```python
from build123d import *

# Parameters (mm, degrees)
F0_R     = 1.5
F0_R_2   = 1.65
F0_R_3   = 5
F1_DEPTH = 3
F2_R     = 5


with BuildPart() as f1:
    # F0 (on Top) → F1 (new body)
    with BuildSketch(Plane.XY):
        with BuildLine():
            add(Edge.make_bspline(
                [(-52.118164, 69.593788), (-40.285984, 48.277058), (-22.257566, 29.243172), (0, 20)],
                knots=[9.256523, 9.256523, 9.256523, 9.256523, 80.865454, 80.865454, 80.865454, 80.865454], degree=3))
            ThreePointArc((-52.118164, 69.593788), (-51.973476, 68.388311), (-51.925144, 67.175144))
            ThreePointArc((-51.925144, 67.175144), (-57.28378, 55.568103), (-69.593788, 52.118164))
            add(Edge.make_bspline(
                [(-69.593788, 52.118164), (-48.277057, 40.285984), (-29.243172, 22.257566), (-20, 0)],
                knots=[9.256523, 9.256523, 9.256523, 9.256523, 80.865454, 80.865454, 80.865454, 80.865454], degree=3))
            Line((-20, 0), (0, 0))
            Line((0, 0), (0, 20))
        make_face()
        with Locations((-18, 6.25)):
            Circle(F0_R, mode=Mode.SUBTRACT)
        with Locations((-7.5, 7.5)):
            Circle(F0_R, mode=Mode.SUBTRACT)
        with Locations((-6.25, 18)):
            Circle(F0_R, mode=Mode.SUBTRACT)
        with BuildLine():
            add(Edge.make_bspline(
                [(-56.391766, 77.958523), (-55.0736, 75.142944), (-53.64765, 72.349293), (-52.118164, 69.593788)],
                knots=[0, 0, 0, 0, 9.256523, 9.256523, 9.256523, 9.256523], degree=3))
            ThreePointArc((-56.391766, 77.958523), (-77.958523, 77.958523), (-77.958523, 56.391766))
            add(Edge.make_bspline(
                [(-77.958523, 56.391766), (-75.142944, 55.0736), (-72.349293, 53.647649), (-69.593788, 52.118164)],
                knots=[0, 0, 0, 0, 9.256523, 9.256523, 9.256523, 9.256523], degree=3))
            ThreePointArc((-69.593788, 52.118164), (-57.28378, 55.568103), (-51.925144, 67.175144))
            ThreePointArc((-51.925144, 67.175144), (-51.973476, 68.388311), (-52.118164, 69.593788))
        make_face()
        with Locations((-67.175142, 57.675142)):
            Circle(F0_R_2, mode=Mode.SUBTRACT)
        with Locations((-75.175142, 67.175142)):
            Circle(F0_R_2, mode=Mode.SUBTRACT)
        with Locations((-67.175142, 67.175142)):
            Circle(F0_R_3, mode=Mode.SUBTRACT)
        with Locations((-67.175142, 76.675142)):
            Circle(F0_R_2, mode=Mode.SUBTRACT)
        with Locations((-59.175142, 67.175142)):
            Circle(F0_R_2, mode=Mode.SUBTRACT)
    extrude(amount=F1_DEPTH)

    # F2
    f2_edges = [f1.edges().sort_by_distance(p)[0] for p in [
        (-56.391766, 77.958523, 1.5),
        (-77.958523, 56.391766, 1.5),
    ]]
    fillet(f2_edges, radius=F2_R)


solid = f1.part
```
Model file for the job. Use its own axes, mm. Give positions to 0.01 mm unless a question says otherwise; leave off trailing zeros.
1) Pin check, flat tips, straight feed: pin 1 (4 mm diameter, centred on x = -67.18, y = 57.68, fed in from +Z); pin 2 (1.5 mm diameter, centred on x = -52.5, z = 1, fed in from -Y); pin 3 (1.5 mm diameter, centred on x = -47.5, z = 0.5, fed in from -Y). Stop position of each tip, or through.
2) Saw through at A-A, the plane z = 2.2. Count the separate pieces of the cut face and the enclosed holes in it, then the cut area to 3 significant figures.
3) Mould opens along X. For faces 1 (the cylindrical face through (-68.485, 56.671, 1.479)), 2 (the flat face through (-41, 41, 3)), 3 (the flat face through (0, 10, 1)), 4 (the cylindrical face through (-77.73, 78.18, 1.48)) say: +X half, -X half, draft (parallel to the pull), parting line (faces both ways), or undercut.
4) Wall check: probe 1 along Y at (x, z) = (-58, 2.85); probe 2 along Y at (x, z) = (-74.5, 2.05); probe 3 along X at (y, z) = (76, 0.95). Give the ranges that are in metal, low to high.
Computed:
1. pin 1: stops at z = 3
1. pin 2: stops at y = 40.26
1. pin 3: stops at y = 36.1
2. separate pieces: 1
2. enclosed holes: 8
2. area: 2,000 mm2
3. face 1: undercut
3. face 2: draft
3. face 3: +X half
3. face 4: parting line
4. probe 1: y = 44.9 to 66.02, 68.33 to 79.36
4. probe 2: y = 54.71 to 65.67, 68.68 to 80.55
4. probe 3: x = -79.61 to -68.68, -65.67 to -55.46
